Autodesk Inventor part; units mm, degrees
ref_plane "YZ Plane" through (0, 0, 0) normal (1, 0, 0) x (0, 1, 0)
ref_plane "XZ Plane" through (0, 0, 0) normal (0, 1, 0) x (-1, 0, 0)
ref_plane "XY Plane" through (0, 0, 0) normal (0, 0, 1) x (1, 0, 0)
sketch "Sketch1" plane through (0, 0, 0) normal (0, 0, 1) x (1, 0, 0)
  line L0 (0, 0) -> (400, 0)
  line L1 (400, 0) -> (400, 250)
  line L2 (400, 250) -> (0, 250)
  line L3 (0, 250) -> (0, 0)
  dimension "d0" = 400
  dimension "d1" = 250
extrude "Extrusion1" add sketch "Sketch1" along normal mid plane 250
sketch "Sketch2" plane through (0, 0, 0) normal (0, 0, 1) x (1, 0, 0)
  line L0 (400, 0) -> (400, 250)
  line L1 (400, 225) -> (275, 250)
  line L2 (400, 250) -> (0, 250)
  line L3 (275, 250) -> (400, 250)
  line L4 (400, 225) -> (400, 250)
  line L5 (400, 25) -> (275, 0)
  line L6 (0, 0) -> (400, 0)
  line L7 (225, 250) -> (0, 200)
  line L8 (0, 250) -> (0, 0)
  line L9 (225, 0) -> (0, 50)
  line L10 (400, 25) -> (400, 0)
  line L11 (275, 0) -> (400, 0)
  line L12 (225, 0) -> (0, 0)
  line L13 (0, 0) -> (0, 50)
  line L14 (0, 200) -> (0, 250)
  line L15 (225, 250) -> (0, 250)
  dimension "d4" = 25
  dimension "d5" = 125
  dimension "d6" = 25
  dimension "d7" = 125
  dimension "d8" = 50
  dimension "d9" = 50
  dimension "d10" = 50
  dimension "d11" = 50
extrude "Extrusion2" cut sketch "Sketch2" along normal through all both and the other way through all contours L6 L5 L0 | L1 L2 L0 | L6 L8 L9 | L7 L8 L2
sketch "Sketch3" plane through (0, 0, 0) normal (0, 1, 0) x (-1, 0, 0)
  line L0 (-275, -125) -> (-400, -125)
  line L1 (-400, -125) -> (-400, -100)
  line L2 (-400, -100) -> (-275, -125)
  line L3 (-275, 125) -> (-400, 125)
  line L4 (-400, 125) -> (-400, 100)
  line L5 (-275, 125) -> (-400, 100)
  line L6 (0, 0) -> (-400, 0) construction
  line L7 (0, 0) -> (0, 125) construction
  line L8 (0, 0) -> (0, -125) construction
  dimension "d28" = 25
  dimension "d29" = 25
  dimension "d32" = 400
  dimension "d33" = 100
  dimension "d34" = 100
  dimension "d35" = 125
  dimension "d36" = 125
  dimension "d37" = 125
  dimension "d38" = 125
  dimension "d39" = 400
  dimension "d40" = 400
extrude "Extrusion3" cut sketch "Sketch3" along normal through all
sketch "Sketch4" plane through (0, 0, 0) normal (0, 1, 0) x (-1, 0, 0)
  line L0 (0, -125) -> (-400, -125)
  line L1 (-225, -125) -> (0, -125)
  line L2 (0, -125) -> (0, -100)
  line L3 (0, -100) -> (-225, -125)
  line L4 (-225, 125) -> (0, 125)
  line L5 (-225, 125) -> (0, 125)
  line L6 (0, 125) -> (0, 100)
  line L7 (0, 100) -> (-225, 125)
  point P0 (0, 0)
  point P1 (-275, -125)
  dimension "d18" = 25
  dimension "d19" = 25
extrude "Extrusion4" cut sketch "Sketch4" along normal through all
chamfer "Chamfer1" distance 20 angle 45 4 edges at (0, 125, -100) (0, 125, 100) (0, 200, 0) (0, 50, 0)
chamfer "Chamfer2" distance 20 angle 45 4 edges at (400, 225, 0) (400, 125, -100) (400, 125, 100) (400, 25, 0)
properties part number "Scorpion Body"
Geometry check sheet. Reference: the model listing, model coordinates, mm. Round coordinates to 2 decimals unless told otherwise and drop trailing zeros. Order: outer loops, then holes, each group sorted by start corner. A loop starts at its lowest first (then second) coordinate and runs counter-clockwise, first axis right, second up. Notation, with made-up numbers: (6, -1) -> (30, -1) arc R5 cw to (30, 3) -> close; hole circle Ø11 at (78, -8). An arc over 180 degrees is marked (long way). Use one line per item in the form item = value.
1. Cross-section at C-C, the plane x = 298. Enter the section's corners in (y, z).
Working result:
outline = (4.6, -120.4) -> (245.4, -120.4) -> (245.4, 120.4) -> (4.6, 120.4) -> close
2. Cross-section at D-D, the plane x = 47.5. Enter the section's corners in (y, z).
Working result:
outline = (39.44, -105.28) -> (210.56, -105.28) -> (210.56, 105.28) -> (39.44, 105.28) -> close
3. Cross-section at A-A, the plane y = 148. Enter the section's corners in (x, z).
Working result:
outline = (0, -80) -> (19.88, -102.21) -> (225, -125) -> (275, -125) -> (380.39, -103.92) -> (400, -80) -> (400, 80) -> (380.39, 103.92) -> (275, 125) -> (225, 125) -> (19.88, 102.21) -> (0, 80) -> close
4. Scan lines: line 1 along Y through (x, z) = (66, 61); line 2 along Z through (x, y) = (324, 203.5); line 3 along X through (y, z) = (63.5, 21). Record each from-to range of solid material in increasing order. Write a range as from..to.
Working result:
line_1 = 35.33..214.67
line_2 = -115.2..115.2
line_3 = 5.21..400
5. Go/stop test with flat-tipped pins: pin 1 (4 mm diameter, centred on x = 102.5, z = -25, fed in from -Y); pin 2 (10 mm diameter, centred on x = 288.5, z = -59.5, fed in from +Y); pin 3 (2 mm diameter, centred on y = 221.5, z = -65.5, fed in from +X); pin 4 (1.5 mm diameter, centred on x = 233, z = 85, fed in from -Y). Record where each tip stops, or that it passes through.
Working result:
pin_1 = 26.78
pin_2 = 248.3
pin_3 = 387.29
pin_4 = 0
6. Cross-section at B-B, the plane z = -60. Enter the section's corners in (x, y), plus the area to 3 significant figures.
Working result:
outline = (0, 70) -> (19.52, 45.66) -> (225, 0) -> (275, 0) -> (380.39, 21.08) -> (400, 45) -> (400, 205) -> (380.39, 228.92) -> (275, 250) -> (225, 250) -> (19.52, 204.34) -> (0, 180) -> close
area = 84,800 mm^2
